Geometry check sheet. Reference: the model listing, model coordinates, mm. Face numbers are marked on the shaded views. A direction names the side the tool comes from. Coordinates: 2 decimals unless noted, no trailing zeros. Loops run counter-clockwise (first coordinate to the right, second up) from the corner with the lowest first, then second, coordinate; pieces in that order, holes last. Notation, with made-up numbers: M 16.5,-20 L 73.5,-20 A30 cw 73.5,3 Z; hole C -37,70 d6. An arc over 180 degrees is marked long. Use CSV: the item, a comma, the result in double quotes.
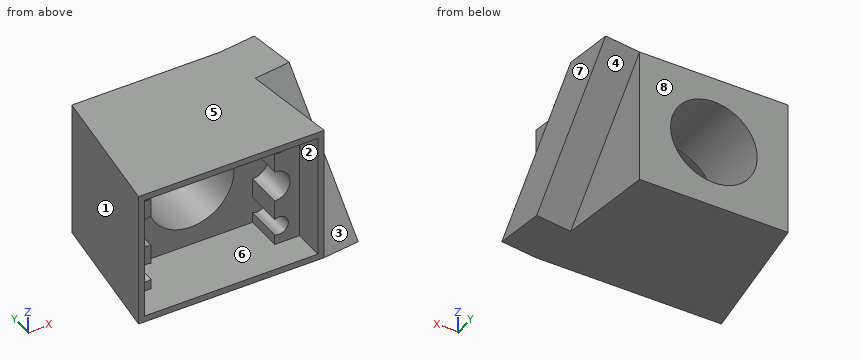
```python
from build123d import *

# Parameters (mm, degrees)
F0_W     = 30
F0_H     = 22
F1_DEPTH = 23
F2_DEPTH = 18
F0_R     = 7
F3_DEPTH = 12
F4_DEPTH = 12
F6_DEPTH = 25
F8_DEPTH = 6


with BuildPart() as f1:
    # F0 (on Front) → F1 (new body)
    with BuildSketch(Plane.XZ):
        with Locations((0, -11)):
            Rectangle(F0_W, F0_H)
        Polygon((-14, -21), (-14, -1), (-10, -1), (10, -1), (14, -1), (14, -21), (10, -21), (-10, -21), align=None, mode=Mode.SUBTRACT)
    extrude(amount=F1_DEPTH)

    # F0 (on Front) → F2 (join)
    with BuildSketch(Plane.XZ):
        with BuildLine():
            Line((-10, -1), (-14, -1))
            Line((-14, -1), (-14, -21))
            Line((-14, -21), (-10, -21))
            Line((-10, -21), (-10, -19.3266499161))
            ThreePointArc((-10, -19.3266499161), (-12.2, -18), (-10, -16.6733500839))
            Line((-10, -16.6733500839), (-10, -13.5))
            ThreePointArc((-10, -13.5), (-12.5, -11), (-10, -8.5))
            Line((-10, -8.5), (-10, -5.3266499161))
            ThreePointArc((-10, -5.3266499161), (-12.2, -4), (-10, -2.6733500839))
            Line((-10, -2.6733500839), (-10, -1))
        make_face()
        with BuildLine():
            Line((14, -1), (10, -1))
            Line((10, -1), (10, -2.6733500839))
            ThreePointArc((10, -2.6733500839), (11.4745966692, -2.7154767421), (12.2, -4))
            ThreePointArc((12.2, -4), (11.4745966692, -5.2845232579), (10, -5.3266499161))
            Line((10, -5.3266499161), (10, -8.5))
            ThreePointArc((10, -8.5), (12.5, -11), (10, -13.5))
            Line((10, -13.5), (10, -16.6733500839))
            ThreePointArc((10, -16.6733500839), (11.4745966692, -16.7154767421), (12.2, -18))
            ThreePointArc((12.2, -18), (11.4745966692, -19.2845232579), (10, -19.3266499161))
            Line((10, -19.3266499161), (10, -21))
            Line((10, -21), (14, -21))
            Line((14, -21), (14, -1))
        make_face()
    extrude(amount=F2_DEPTH)

    # F0 (on Front) → F3 (join)
    with BuildSketch(Plane.XZ):
        with BuildLine():
            Line((10, -1), (-10, -1))
            Line((-10, -1), (-10, -2.6733500839))
            ThreePointArc((-10, -2.6733500839), (-9.4154767421, -3.2254033308), (-9.2, -4))
            ThreePointArc((-9.2, -4), (-9.4154767421, -4.7745966692), (-10, -5.3266499161))
            Line((-10, -5.3266499161), (-10, -8.5))
            ThreePointArc((-10, -8.5), (-12.5, -11), (-10, -13.5))
            Line((-10, -13.5), (-10, -16.6733500839))
            ThreePointArc((-10, -16.6733500839), (-9.4154767421, -17.2254033308), (-9.2, -18))
            ThreePointArc((-9.2, -18), (-9.4154767421, -18.7745966692), (-10, -19.3266499161))
            Line((-10, -19.3266499161), (-10, -21))
            Line((-10, -21), (10, -21))
            Line((10, -21), (10, -19.3266499161))
            ThreePointArc((10, -19.3266499161), (9.2, -18), (10, -16.6733500839))
            Line((10, -16.6733500839), (10, -13.5))
            ThreePointArc((10, -13.5), (12.5, -11), (10, -8.5))
            Line((10, -8.5), (10, -5.3266499161))
            ThreePointArc((10, -5.3266499161), (9.2, -4), (10, -2.6733500839))
            Line((10, -2.6733500839), (10, -1))
        make_face()
        with Locations((0, -11)):
            Circle(F0_R, mode=Mode.SUBTRACT)
    extrude(amount=F3_DEPTH)

    # F0 (on Front) → F4 (join)
    with BuildSketch(Plane.XZ):
        with BuildLine():
            ThreePointArc((-9.2, -4), (-9.4154767421, -3.2254033308), (-10, -2.6733500839))
            ThreePointArc((-10, -2.6733500839), (-12.2, -4), (-10, -5.3266499161))
            ThreePointArc((-10, -5.3266499161), (-9.4154767421, -4.7745966692), (-9.2, -4))
        make_face()
        with BuildLine():
            ThreePointArc((12.2, -4), (11.4745966692, -2.7154767421), (10, -2.6733500839))
            ThreePointArc((10, -2.6733500839), (9.2, -4), (10, -5.3266499161))
            ThreePointArc((10, -5.3266499161), (11.4745966692, -5.2845232579), (12.2, -4))
        make_face()
        with BuildLine():
            ThreePointArc((10, -16.6733500839), (9.2, -18), (10, -19.3266499161))
            ThreePointArc((10, -19.3266499161), (11.4745966692, -19.2845232579), (12.2, -18))
            ThreePointArc((12.2, -18), (11.4745966692, -16.7154767421), (10, -16.6733500839))
        make_face()
        with BuildLine():
            ThreePointArc((-10, -16.6733500839), (-12.2, -18), (-10, -19.3266499161))
            ThreePointArc((-10, -19.3266499161), (-9.4154767421, -18.7745966692), (-9.2, -18))
            ThreePointArc((-9.2, -18), (-9.4154767421, -17.2254033308), (-10, -16.6733500839))
        make_face()
    extrude(amount=F4_DEPTH)

    # F5 (on face) → F6 (cut)
    with BuildSketch(Plane.XY):
        Polygon((-15, -23), (-12, 0), (-15, 0), align=None)
        Polygon((15, 0), (12, 0), (15, -23), align=None)
    extrude(amount=-F6_DEPTH, mode=Mode.SUBTRACT)

    # F7 (on face) → F8 (join)
    with BuildSketch(Plane(origin=(11.7992565056, 1.5390334572, 0), x_dir=(-0.1293391841, 0.9916004112, 0), z_dir=(0.9916004112, 0.1293391841, 0))):
        Polygon((-1.5520702088, 0), (-9.3423313777, 0), (-24.7468972183, -22), (-16.9566360494, -22), align=None)
    extrude(amount=F8_DEPTH)


solid = f1.part
```
1. Thickness scan on line 1 (Z direction, x = -6.5, y = -15); line 2 (Z direction, x = -10.7, y = -13.9); line 3 (Y direction, x = 7, z = -15). Record the ranges inside material, lowest first. Write a range as [from, to].
The answers:
line 1,"[-22, -21], [-1, 0]"
line 2,"[-22, -19.5], [-16.5, -13.4], [-8.6, -5.5], [-2.5, 0]"
line 3,"[-12, 0]"
2. Section check A-A, the plane z = -16. Record the cut outline in (x, y).
The answers:
outline,"M -15,-23 L -14,-23 L -14,-18 L -10,-18 L -10,-12 L -4.9,-12 L -4.9,0 L -12,0 Z; M 4.9,-12 L 10,-12 L 10,-18 L 14,-18 L 14,-23 L 15,-23 L 14.46,-18.83 L 20.41,-18.06 L 19.4,-10.33 L 13.45,-11.11 L 12,0 L 4.9,0 Z"
3. Section check D-D, the plane x = -10.7. Record the cut outline in (y, z), plus the area to 3 significant figures.
The answers:
outline,"M -23,-22 L 0,-22 L 0,0 L -23,0 L -23,-1 L -18,-1 L -18,-2.5 L -12,-2.5 L -12,-5.5 L -18,-5.5 L -18,-8.6 L -12,-8.6 L -12,-13.4 L -18,-13.4 L -18,-16.5 L -12,-16.5 L -12,-19.5 L -18,-19.5 L -18,-21 L -23,-21 Z"
area,"341 mm^2"
4. Set-up check for the marked faces 1, 2, 3, 4 and 5: record each of +Z, -Z, +X, -X, +Y, -Y from which the full face is reachable in a straight line by a thin tool's end or side.
The answers:
face 1,"+Z, -Z, -X, +Y"
face 2,"-Y"
face 3,"+Z, +X"
face 4,"-Z, +Y"
face 5,"+Z, +X, -X, +Y, -Y"
5. Gauge pin test, flat ends, axial feed: P1, Ø1, axis at y = -14, z = -7, coming from the +X side; P2, Ø1.8, axis at y = -16, z = -20, coming from the -X side; P3, Ø2, axis at x = 17, z = -12, coming from the +Y side. Record the tip position at first contact, or that the pin passes through.
The answers:
P1,"x = 13.89"
P2,"x = -14.2"
P3,"y = -7.1"
6. Release check for a two-part mould opening along X. For the marked faces 6, 7 and 8 record: +X half, -X half, draft (parallel to the pull), parting line (faces both ways), or undercut.
The answers:
face 6,"undercut"
face 7,"+X half"
face 8,"draft"
7. Section check C-C, the plane y = -13.5. Record the cut outline in (x, z).
The answers:
outline,"M -13.76,-22 L 13.76,-22 L 13.76,-19.44 L 19.81,-20.56 L 19.81,-9.44 L 13.76,-8.32 L 13.76,0 L -13.76,0 Z; hole M -10,-21 L 10,-21 L 10,-19.33 A1.5 ccw long 10,-16.67 L 10,-13.5 A2.5 ccw 10,-8.5 L 10,-5.33 A1.5 ccw long 10,-2.67 L 10,-1 L -10,-1 L -10,-2.67 A1.5 ccw long -10,-5.33 L -10,-8.5 A2.5 ccw -10,-13.5 L -10,-16.67 A1.5 ccw long -10,-19.33 Z"
8. Section check B-B, the plane x = 3. Record the cut outline in (y, z).
The answers:
outline,"M -23,-22 L 0,-22 L 0,-17.32 L -12,-17.32 L -12,-21 L -23,-21 Z; M -23,-1 L -12,-1 L -12,-4.68 L 0,-4.68 L 0,0 L -23,0 Z"
